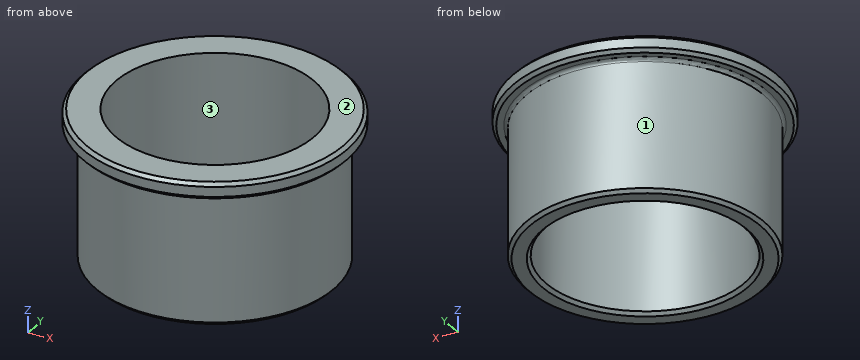
```python
from build123d import *

# Parameters (mm, degrees)
FILLET1_R     = 0.5
CHAMFER1_SIZE = 0.5


with BuildPart() as part:
    # Sketch1 → Revolve1 (revolve)
    with BuildSketch(Plane(origin=(0, 0, 0), x_dir=(0, 0, -1), z_dir=(1, 0, 0))):
        Polygon((0, 15), (0, 20), (2.5, 20), (2.5, 18), (22.5, 18), (22.5, 15), align=None)
    revolve(axis=Axis((0, 0, 38.983478261), (0, 0, -1)))

    # Fillet1
    fillet1_edges = [part.edges().sort_by_distance(p)[0] for p in [
        (0, -18, -2.5),
    ]]
    fillet(fillet1_edges, radius=FILLET1_R)

    # Chamfer1
    chamfer1_edges = [part.edges().sort_by_distance(p)[0] for p in [
        (0, -20, -2.5),
        (0, -20, 0),
        (0, -18, -22.5),
        (0, -15, -22.5),
    ]]
    chamfer(chamfer1_edges, length=CHAMFER1_SIZE)


solid = part.part
```
Build history of the part. All positions in model axes, mm. Face numbers are marked on the shaded views. Round coordinates to 2 decimals unless told otherwise and drop trailing zeros. Loops run counter-clockwise (first coordinate to the right, second up) from the corner with the lowest first, then second, coordinate; pieces in that order, holes last.
Item 1: Saw through at A-A (y = 0). List the corners of the cut face in (x, z), then the cut area to 3 significant figures.
Item 2: Two-plate mould, pull along Y, no slides. Class the marked faces 1, 2 and 3: released by +Y, released by -Y, zero draft, split by the parting line, or undercut.
Item 3: Pin check, flat tips, straight feed: P1, Ø10, axis at y = -13.5, z = -8, coming from the -X side; P2, Ø1.5, axis at x = 16, z = -15.5, coming from the -Y side; P3, Ø10, axis at y = 1, z = -18.5, coming from the -X side. Stop position of each tip, or through.
Item 4: Saw through at C-C (z = -11). List the corners of the cut face in (x, y).
Item 5: Drill centre lines: line 1 along X through (y, z) = (0, -7.75); line 2 along Y through (x, z) = (8.5, -8.5); line 3 along Y through (x, z) = (9, -16.5). Where is each one in solid material? Low to high.
Worked answers:
1. outline: (-20, -2) - (-19.5, -2.5) - (-18.5, -2.5) arc R0.5 cw to (-18, -3) - (-18, -22) - (-17.5, -22.5) - (-15.5, -22.5) - (-15, -22) - (-15, 0) - (-19.5, 0) - (-20, -0.5) - close; (15, -22) - (15.5, -22.5) - (17.5, -22.5) - (18, -22) - (18, -3) arc R0.5 cw to (18.5, -2.5) - (19.5, -2.5) - (20, -2) - (20, -0.5) - (19.5, 0) - (15, 0) - close
1. area: 144 mm2
2. face 1: split by the parting line
2. face 2: zero draft
2. face 3: undercut
3. P1: stops at x = -15.87
3. P2: stops at y = -9.56
3. P3: stops at x = -18
4. outline: circle Ø36 at (0, 0); hole circle Ø30 at (0, 0)
5. line 1: x = -18 to -15, 15 to 18
5. line 2: y = -15.87 to -12.36, 12.36 to 15.87
5. line 3: y = -15.59 to -12, 12 to 15.59
